```python
from build123d import *

# Parameters (mm, degrees)
F0_W     = 98.044
F0_H     = 241.3
F1_DEPTH = 35.56
F2_R     = 2
F3_DEPTH = 9.525


with BuildPart() as f1:
    # F0 (on Top) → F1 (new body)
    with BuildSketch(Plane.XY):
        with Locations((49.022, 120.65)):
            Rectangle(F0_W, F0_H)
    extrude(amount=F1_DEPTH)

    # F2 (on face) → F3 (cut)
    with BuildSketch(Plane.XY.offset(35.56)):
        with Locations((9.525, 12.7)):
            Circle(F2_R)
        with Locations((9.525, 19.05)):
            Circle(F2_R)
        with Locations((9.525, 25.4)):
            Circle(F2_R)
        with Locations((9.525, 31.75)):
            Circle(F2_R)
        with Locations((9.525, 38.1)):
            Circle(F2_R)
        with Locations((22.225, 38.1)):
            Circle(F2_R)
        with Locations((22.225, 31.75)):
            Circle(F2_R)
        with Locations((22.225, 25.4)):
            Circle(F2_R)
        with Locations((22.225, 19.05)):
            Circle(F2_R)
        with Locations((22.225, 12.7)):
            Circle(F2_R)
        with Locations((9.525, 76.2)):
            Circle(F2_R)
        with Locations((9.525, 69.85)):
            Circle(F2_R)
        with Locations((9.525, 63.5)):
            Circle(F2_R)
        with Locations((9.525, 57.15)):
            Circle(F2_R)
        with Locations((9.525, 50.8)):
            Circle(F2_R)
        with Locations((22.225, 50.8)):
            Circle(F2_R)
        with Locations((22.225, 57.15)):
            Circle(F2_R)
        with Locations((22.225, 63.5)):
            Circle(F2_R)
        with Locations((22.225, 76.2)):
            Circle(F2_R)
        with Locations((22.225, 69.85)):
            Circle(F2_R)
        with Locations((9.525, 114.3)):
            Circle(F2_R)
        with Locations((9.525, 107.95)):
            Circle(F2_R)
        with Locations((9.525, 101.6)):
            Circle(F2_R)
        with Locations((9.525, 95.25)):
            Circle(F2_R)
        with Locations((9.525, 88.9)):
            Circle(F2_R)
        with Locations((22.225, 88.9)):
            Circle(F2_R)
        with Locations((22.225, 95.25)):
            Circle(F2_R)
        with Locations((22.225, 101.6)):
            Circle(F2_R)
        with Locations((22.225, 114.3)):
            Circle(F2_R)
        with Locations((22.225, 107.95)):
            Circle(F2_R)
        with Locations((9.525, 152.4)):
            Circle(F2_R)
        with Locations((9.525, 146.05)):
            Circle(F2_R)
        with Locations((9.525, 139.7)):
            Circle(F2_R)
        with Locations((9.525, 133.35)):
            Circle(F2_R)
        with Locations((9.525, 127)):
            Circle(F2_R)
        with Locations((22.225, 127)):
            Circle(F2_R)
        with Locations((22.225, 133.35)):
            Circle(F2_R)
        with Locations((22.225, 139.7)):
            Circle(F2_R)
        with Locations((22.225, 152.4)):
            Circle(F2_R)
        with Locations((22.225, 146.05)):
            Circle(F2_R)
        with Locations((9.525, 190.5)):
            Circle(F2_R)
        with Locations((9.525, 184.15)):
            Circle(F2_R)
        with Locations((9.525, 177.8)):
            Circle(F2_R)
        with Locations((9.525, 171.45)):
            Circle(F2_R)
        with Locations((9.525, 165.1)):
            Circle(F2_R)
        with Locations((22.225, 165.1)):
            Circle(F2_R)
        with Locations((22.225, 171.45)):
            Circle(F2_R)
        with Locations((22.225, 177.8)):
            Circle(F2_R)
        with Locations((22.225, 190.5)):
            Circle(F2_R)
        with Locations((22.225, 184.15)):
            Circle(F2_R)
        with Locations((9.525, 228.6)):
            Circle(F2_R)
        with Locations((9.525, 222.25)):
            Circle(F2_R)
        with Locations((9.525, 215.9)):
            Circle(F2_R)
        with Locations((9.525, 209.55)):
            Circle(F2_R)
        with Locations((9.525, 203.2)):
            Circle(F2_R)
        with Locations((22.225, 203.2)):
            Circle(F2_R)
        with Locations((22.225, 209.55)):
            Circle(F2_R)
        with Locations((22.225, 215.9)):
            Circle(F2_R)
        with Locations((22.225, 228.6)):
            Circle(F2_R)
        with Locations((22.225, 222.25)):
            Circle(F2_R)
    extrude(amount=-F3_DEPTH, mode=Mode.SUBTRACT)


solid = f1.part
```
CAD build for the part. Positions are in the model's coordinates, mm. Coordinates: 2 decimals unless noted, no trailing zeros. Use one line per item in the form item = value. Start each with the question number.
1) Drill centre line: L1, parallel to X at y = 133.35, z = 29.5 (3 decimals). Where is it in solid material? Low to high. Write a range as [from, to].
2) Drop flat-ended pins along their axis: pin 1 (5 mm diameter, centred on y = 195.5, z = 32, fed in from -X); pin 2 (2 mm diameter, centred on x = 9.5, y = 26, fed in from +Z) (3 decimals). Give the stop position or say it passes through.
3) Pull direction Y, two halves, no side cores. Call faces 1 (the flat face through (48, 0, 18)), 2 (the flat face through (9, 210, 26.035)), 3 (the flat face through (22, 171, 26.035)): +Y half, -Y half, draft (parallel to the pull), parting line (faces both ways), or undercut.
Entries:
q1.L1 = [0, 7.525], [11.525, 20.225], [24.225, 98.044]
q2.pin_1 = 0
q2.pin_2 = 26.035
q3.face_1 = -Y half
q3.face_2 = undercut
q3.face_3 = undercut
